The model under review builds one solid part; all positions refer to its coordinate system, in mm. A direction names the side the tool comes from. Give positions to 0.01 mm unless a question says otherwise; leave off trailing zeros. Order: outer loops, then holes, each group sorted by start corner. A loop starts at its lowest first (then second) coordinate and runs counter-clockwise, first axis right, second up. Notation, with made-up numbers: M 25.5,35.25 L 53.5,35.25 A13 cw 53.5,52.25 Z; hole C 13,10.25 d1. An arc over 180 degrees is marked long. One line per question, with ' | ' between items. Start each with the question number.
1. Wall thickness on L1, parallel to X at y = 2, z = 0.35; L2, parallel to Y at x = 12.5, z = 0.65; L3, parallel to Z at x = 4, y = 8: over which ranges is each line inside the solid? List them lowest first.
2. The part is to be moulded in two halves that separate along Y. For faces 1 (the face through (-0.3, -6, 0.5)), 2 (the face through (0, 0, 1)), 3 (the face through (-0.126, 6.538, 1.177)), say which applies: +Y half, -Y half, draft (parallel to the pull), parting line (faces both ways), or undercut.
3. We need section B-B on x = -12.5. Write out the cut boundary in (y, z).
4. We need section D-D on x = 16. Write out the cut boundary in (y, z).
5. For faces 4 (the face through (10, 0.1, 0.5)), 5 (the face through (0, 0, 0)), list the 3-axis set-ups (+Z, -Z, +X, -X, +Y, -Y) from which the entire face can be reached by the end or side of a thin tool; tool diameter is ignored.
6. We need section A-A on y = 0. Write out the cut boundary in (x, z).
7. We need section C-C on z = 2.4. Write out the cut boundary in (x, y).
8. Insertion check: P1, Ø3.5, axis at x = -2, y = -3, coming from the +Z side; P2, Ø1, axis at x = -4.5, y = -2.5, coming from the -Z side; P3, Ø1.1, axis at x = 6.5, z = 0.5, coming from the +Y side. Each pin has a flat end and moves straight along its axis. Give the tip position at first contact, or say it passes through.
```python
from build123d import *

# Parameters (mm, degrees)
SKETCH_1_W      = 38
SKETCH_1_H      = 12
SKETCH_1_R      = 2.5
EXTRUDE_1_DEPTH = 1
SKETCH_3_R      = 2.50184692
SKETCH_3_R_2    = 1.5
EXTRUDE_2_DEPTH = 18


with BuildPart() as part:
    # 草图1 → 凸台-拉伸1 (new body)
    with BuildSketch(Plane.XY):
        Rectangle(SKETCH_1_W, SKETCH_1_H)
        with Locations((12.5, 0)):
            Circle(SKETCH_1_R, mode=Mode.SUBTRACT)
        with Locations((-12.5, 0)):
            Circle(SKETCH_1_R, mode=Mode.SUBTRACT)
    extrude(amount=EXTRUDE_1_DEPTH)

    # 草图3 → 凸台-拉伸2 (add)
    with BuildSketch(Plane.ZY.offset(9)):
        with Locations((1.50184692, 8.00184692)):
            Circle(SKETCH_3_R)
        with Locations((1.50184692, 8.00184692)):
            Circle(SKETCH_3_R_2, mode=Mode.SUBTRACT)
    extrude(amount=-EXTRUDE_2_DEPTH)


solid = part.part
```
Entries:
1) L1: x = -19 to -14, -11 to 11, 14 to 19 | L2: y = -6 to -2.5, 2.5 to 6 | L3: z = -1 to 0, 3 to 4
2) face 1: -Y half | face 2: draft | face 3: undercut
3) outline: M -6,0 L -2.5,0 L -2.5,1 L -6,1 Z; M 2.5,0 L 6,0 L 6,1 L 2.5,1 Z
4) outline: M -6,0 L 6,0 L 6,1 L -6,1 Z
5) face 4: +Z, -Z | face 5: -Z, +X, -X, -Y
6) outline: M -19,0 L -15,0 L -15,1 L -19,1 Z; M -10,0 L 10,0 L 10,1 L -10,1 Z; M 15,0 L 19,0 L 19,1 L 15,1 Z
7) outline: M -9,5.67 L 9,5.67 L 9,6.8 L -9,6.8 Z; M -9,9.2 L 9,9.2 L 9,10.34 L -9,10.34 Z
8) P1: stops at z = 1 | P2: stops at z = 0 | P3: stops at y = 10.46
